Print and shaded views of the part. All mm, measured from the part's lowest x, y and z. Round coordinates to 2 decimals unless told otherwise and drop trailing zeros. Write each loop counter-clockwise with the first axis right and the second up, starting at its lowest first coordinate (ties: lowest second). Pieces come first, ordered by that corner, then holes. Notation, with made-up numbers: (50.25, 78.25) - (64.25, 78.25) arc R20 cw to (64.25, 107.25) - close; hole circle Ø6 at (38.5, 47). An arc over 180 degrees is marked (long way). One line per item, written item: value.
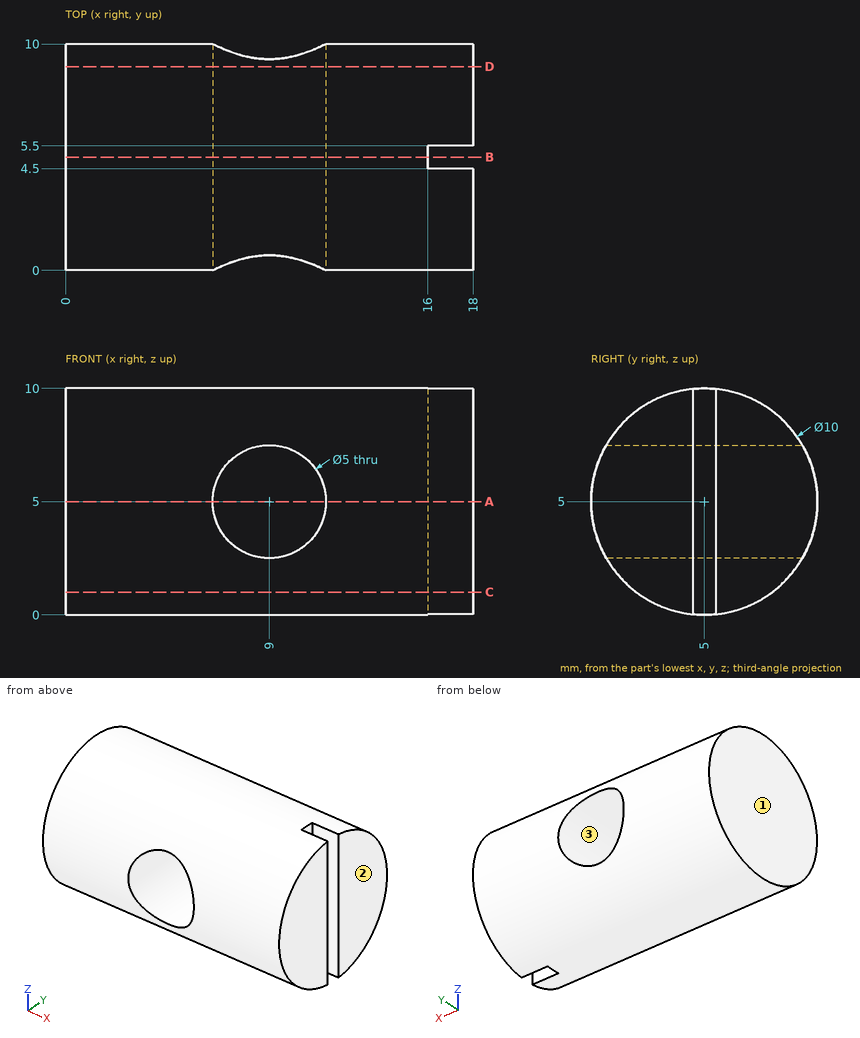
1. Drop flat-ended pins along their axis: pin 1 (1.6 mm diameter, centred on x = 17, z = 3, fed in from -Y); pin 2 (1.5 mm diameter, centred on x = 15.5, y = 1.5, fed in from +Z); pin 3 (2 mm diameter, centred on x = 16.5, z = 4.5, fed in from +Y); pin 4 (2 mm diameter, centred on x = 12, z = 2.5, fed in from +Y). Give the stop position or say it passes through.
Report:
pin 1: y = 0.15
pin 2: z = 9.18
pin 3: y = 10
pin 4: y = 9.77
2. Mould opens along X. For the marked faces 1, 2 and 3 say: released by +X, released by -X, zero draft, split by the parting line, or undercut.
Report:
face 1: released by -X
face 2: released by +X
face 3: undercut
3. Band-saw the part on A-A on z = 5. Write the cut outline in (x, y).
Report:
outline: (0, 0) - (6.5, 0) - (6.5, 10) - (0, 10) - close; (11.5, 0) - (18, 0) - (18, 4.5) - (16, 4.5) - (16, 5.5) - (18, 5.5) - (18, 10) - (11.5, 10) - close
4. Wall check: probe 1 along X at (y, z) = (5, 5); probe 2 along X at (y, z) = (3.75, 5); probe 3 along Z at (x, y) = (8, 2.75). Give the ranges that are in metal, low to high. Write a range as [from, to].
Report:
probe 1: [0, 6.5], [11.5, 16]
probe 2: [0, 6.5], [11.5, 18]
probe 3: [0.53, 2.71], [7.29, 9.47]
5. Band-saw the part on B-B on y = 5. Write the cut outline in (x, z), plus the area to 3 significant figures.
Report:
outline: (0, 0) - (16, 0) - (16, 10) - (0, 10) - close; hole circle Ø5 at (9, 5)
area: 140 mm²
6. Band-saw the part on D-D on y = 9. Write the cut outline in (x, z).
Report:
outline: (0, 2) - (18, 2) - (18, 8) - (0, 8) - close; hole circle Ø5 at (9, 5)
7. Band-saw the part on C-C on z = 1. Write the cut outline in (x, y).
Report:
outline: (0, 2) - (18, 2) - (18, 4.5) - (16, 4.5) - (16, 5.5) - (18, 5.5) - (18, 8) - (0, 8) - close
